Verification items for the finished model (mm, model axes). Face numbers are marked on the shaded views. A direction names the side the tool comes from. Round coordinates to 2 decimals unless told otherwise and drop trailing zeros. Loops run counter-clockwise (first coordinate to the right, second up) from the corner with the lowest first, then second, coordinate; pieces in that order, holes last. Notation, with made-up numbers: (82.25, 57) -> (88.25, 57) arc R22 ccw to (88.25, 63) -> close; hole circle Ø6 at (63.25, -12). An arc over 180 degrees is marked (long way). Write item = value, one per line.
```python
from build123d import *

# Parameters (mm, degrees)
BASE_FLANGE1_DEPTH      = 0.508
EDGE_FLANGE2_START      = -4.7625
EDGE_FLANGE2_DEPTH      = 9.525
EDGE_FLANGE2_2_DEPTH    = 9.525
EDGE_FLANGE3_START      = -4.7625
EDGE_FLANGE3_DEPTH      = 9.525
EDGE_FLANGE3_2_DEPTH    = 9.525
FILLET1_R               = 3.175
SKETCH17_R              = 1.8415
CUT_EXTRUDE1_DEPTH      = 23.441501951
EDGE_FLANGE4_DEPTH      = 4.445
EDGE_FLANGE4_BEND_DEPTH = 4.445
FILLET2_R               = 1.524
EDGE_FLANGE5_DEPTH      = 2.57875744
EDGE_FLANGE5_BEND_DEPTH = 2.57875744
FILLET3_R               = 0.762


# Read off the part's stored shape, not the designer's step: Edge-Flange2, Edge-Flange3
# Sheet-metal steps are written as plain solids
with BuildPart() as part:
    # Sketch1 → Base-Flange1 (new body)
    with BuildSketch(Plane(origin=(0, 0, 0), x_dir=(1, 0, 0), z_dir=(0, 1, 0))):
        with BuildLine():
            Line((-4.7625, -6.35), (-4.7625, -8.89))
            Line((-4.7625, -8.89), (4.7625, -8.89))
            Line((4.7625, -8.89), (4.7625, -6.35))
            ThreePointArc((4.7625, -6.35), (6.526150521, -4.518104207), (7.62, -2.2225))
            Line((7.62, -2.2225), (7.62, 2.2225))
            ThreePointArc((7.62, 2.2225), (6.526150521, 4.518104207), (4.7625, 6.35))
            Line((4.7625, 6.35), (4.7625, 8.89))
            Line((4.7625, 8.89), (-4.7625, 8.89))
            Line((-4.7625, 8.89), (-4.7625, 6.35))
            ThreePointArc((-4.7625, 6.35), (-6.526150521, 4.518104207), (-7.62, 2.2225))
            Line((-7.62, 2.2225), (-7.62, -2.2225))
            ThreePointArc((-7.62, -2.2225), (-6.526150521, -4.518104207), (-4.7625, -6.35))
        make_face()
    extrude(amount=-BASE_FLANGE1_DEPTH)

    # Edge-Flange2 outline → Edge-Flange2 (cut)
    with BuildSketch(Plane.YZ.offset(EDGE_FLANGE2_START)):
        with BuildLine():
            Line((0, -8.89), (0, -8.708309596))
            ThreePointArc((0, -8.708309596), (-0.373760644, -8.267342948), (-0.508, -7.70508998))
            Line((-0.508, -7.70508998), (-0.508, -8.89))
            Line((-0.508, -8.89), (0, -8.89))
        make_face()
    extrude(amount=EDGE_FLANGE2_DEPTH, mode=Mode.SUBTRACT)

    # Edge-Flange2 2 outline → Edge-Flange2 2 (add)
    with BuildSketch(Plane.YZ.offset(EDGE_FLANGE2_START)):
        with BuildLine():
            ThreePointArc((0, -8.708309596), (0.297808861, -8.869775128), (0.628125963, -8.944953901))
            Line((0.628125963, -8.944953901), (9.360304679, -9.708920547))
            Line((9.360304679, -9.708920547), (9.404579797, -9.20285364))
            Line((9.404579797, -9.20285364), (0.67240108, -8.438886994))
            ThreePointArc((0.67240108, -8.438886994), (0.193521514, -8.202729727), (0, -7.70508998))
            Line((0, -7.70508998), (0, -8.708309596))
        make_face()
    extrude(amount=EDGE_FLANGE2_2_DEPTH)

    # Edge-Flange3 outline → Edge-Flange3 (cut)
    with BuildSketch(Plane.YZ.offset(EDGE_FLANGE3_START)):
        with BuildLine():
            ThreePointArc((-0.508, 7.576201681), (-0.373760644, 8.138454649), (0, 8.579421297))
            Line((0, 8.579421297), (0, 8.89))
            Line((0, 8.89), (-0.508, 8.89))
            Line((-0.508, 8.89), (-0.508, 7.576201681))
        make_face()
    extrude(amount=EDGE_FLANGE3_DEPTH, mode=Mode.SUBTRACT)

    # Edge-Flange3 2 outline → Edge-Flange3 2 (add)
    with BuildSketch(Plane.YZ.offset(EDGE_FLANGE3_START)):
        with BuildLine():
            Line((10.878505399, 7.938254101), (0.845074037, 8.816065602))
            ThreePointArc((0.845074037, 8.816065602), (0.400987593, 8.774698018), (0, 8.579421297))
            Line((0, 8.579421297), (0, 7.576201681))
            ThreePointArc((0, 7.576201681), (0.238960253, 8.119280167), (0.80079892, 8.309998695))
            Line((0.80079892, 8.309998695), (10.834230282, 7.432187195))
            Line((10.834230282, 7.432187195), (10.878505399, 7.938254101))
        make_face()
    extrude(amount=EDGE_FLANGE3_2_DEPTH)

    # Fillet1
    fillet1_edges = [part.edges().sort_by_distance(p)[0] for p in [
        (4.7625, 9.382442238, -9.455887093),
        (-4.7625, 9.382442238, -9.455887093),
        (-4.7625, 10.85636784, 7.685220648),
        (4.7625, 10.85636784, 7.685220648),
    ]]
    fillet(fillet1_edges, radius=FILLET1_R)

    # Sketch17 → Cut-Extrude1 (cut, through all)
    with BuildSketch(Plane(origin=(0, 0.77186615, 8.822470462), x_dir=(1, 0, 0), z_dir=(0, 0.08715574274765484, 0.9961946980917459))):
        with Locations(Location((0, 7.18548753, 0), (0, 0, 270))):
            Circle(SKETCH17_R)
    extrude(amount=-CUT_EXTRUDE1_DEPTH, mode=Mode.SUBTRACT)

    # Edge-Flange4 section (across the edge) → Edge-Flange4 (add)
    with BuildSketch(Plane(origin=(-8.3566, 0, -2.2225), x_dir=(1, 0, 0), z_dir=(0, 0, 1))):
        with BuildLine():
            Line((-0.508, 0.7366), (-0.508, 4.572))
            Line((-0.508, 4.572), (0, 4.572))
            Line((0, 4.572), (0, 0.7366))
            ThreePointArc((0, 0.7366), (0.215745145, 0.215745145), (0.7366, 0))
            Line((0.7366, 0), (0.7366, -0.508))
            ThreePointArc((0.7366, -0.508), (-0.1434651, -0.1434651), (-0.508, 0.7366))
        make_face()
    extrude(amount=EDGE_FLANGE4_DEPTH)

    # Edge-Flange4 section 2 (across the edge) → Edge-Flange4 bend (add)
    with BuildSketch(Plane(origin=(8.3566, 0, 2.2225), x_dir=(-1, 0, 0), z_dir=(0, 0, -1))):
        with BuildLine():
            Line((-0.508, 0.7366), (-0.508, 4.572))
            Line((-0.508, 4.572), (0, 4.572))
            Line((0, 4.572), (0, 0.7366))
            ThreePointArc((0, 0.7366), (0.215745145, 0.215745145), (0.7366, 0))
            Line((0.7366, 0), (0.7366, -0.508))
            ThreePointArc((0.7366, -0.508), (-0.1434651, -0.1434651), (-0.508, 0.7366))
        make_face()
    extrude(amount=EDGE_FLANGE4_BEND_DEPTH)

    # Fillet2
    fillet2_edges = [part.edges().sort_by_distance(p)[0] for p in [
        (-8.6106, 4.572, -2.2225),
        (-8.6106, 4.572, 2.2225),
        (8.6106, 4.572, 2.2225),
        (8.6106, 4.572, -2.2225),
    ]]
    fillet(fillet2_edges, radius=FILLET2_R)

    # Edge-Flange5 section (across the edge) → Edge-Flange5 (add)
    with BuildSketch(Plane(origin=(-5.4991, 5.102367626, 7.933660198), x_dir=(1, 0, 0), z_dir=(0, 0.9961946980917459, -0.08715574274765468))):
        with BuildLine():
            Line((-0.508, 0.7366), (-0.508, 4.064))
            Line((-0.508, 4.064), (0, 4.064))
            Line((0, 4.064), (0, 0.7366))
            ThreePointArc((0, 0.7366), (0.215745145, 0.215745145), (0.7366, 0))
            Line((0.7366, 0), (0.7366, -0.508))
            ThreePointArc((0.7366, -0.508), (-0.1434651, -0.1434651), (-0.508, 0.7366))
        make_face()
    extrude(amount=EDGE_FLANGE5_DEPTH)

    # Edge-Flange5 section 2 (across the edge) → Edge-Flange5 bend (add)
    with BuildSketch(Plane(origin=(5.4991, 7.671312115, 7.708906678), x_dir=(-1, 0, 0), z_dir=(0, -0.9961946980917459, 0.08715574274765468))):
        with BuildLine():
            Line((-0.508, 0.7366), (-0.508, 4.064))
            Line((-0.508, 4.064), (0, 4.064))
            Line((0, 4.064), (0, 0.7366))
            ThreePointArc((0, 0.7366), (0.215745145, 0.215745145), (0.7366, 0))
            Line((0.7366, 0), (0.7366, -0.508))
            ThreePointArc((0.7366, -0.508), (-0.1434651, -0.1434651), (-0.508, 0.7366))
        make_face()
    extrude(amount=EDGE_FLANGE5_BEND_DEPTH)

    # Fillet3
    fillet3_edges = [part.edges().sort_by_distance(p)[0] for p in [
        (-5.7531, 4.748166688, 3.885124945),
        (-5.7531, 7.317111177, 3.660371425),
        (5.7531, 7.317111177, 3.660371425),
        (5.7531, 4.748166688, 3.885124945),
    ]]
    fillet(fillet3_edges, radius=FILLET3_R)


solid = part.part
```
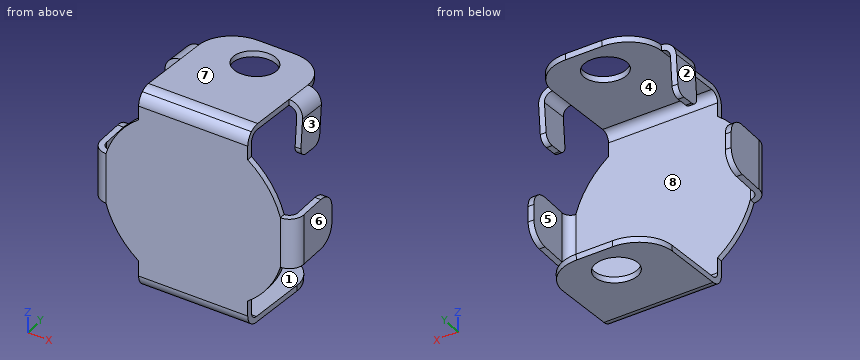
(1) Material ranges on probe 1 along X at (y, z) = (3.25, -0.75); probe 2 along Y at (x, z) = (3.5, -5); probe 3 along X at (y, z) = (6.25, 4.75), recorded low to high. Write a range as from..to.
Filled sheet:
probe_1 = -8.86..-8.36, 8.36..8.86
probe_2 = -0.51..0
probe_3 = -6.01..-5.5, 5.5..6.01
(2) Sectioned sample at B-B, the plane x = -0.75. Record the cut outline in (y, z).
Filled sheet:
outline = (-0.51, -7.71) arc R1.24 ccw to (0.63, -8.94) -> (4.71, -9.3) -> (4.76, -8.8) -> (0.67, -8.44) arc R0.74 cw to (0, -7.71) -> (0, 7.58) arc R0.74 cw to (0.8, 8.31) -> (6.21, 7.84) -> (6.25, 8.34) -> (0.85, 8.82) arc R1.24 ccw to (-0.51, 7.58) -> close; (8.06, -9.6) -> (9.36, -9.71) -> (9.4, -9.2) -> (8.11, -9.09) -> close; (9.56, 7.54) -> (10.83, 7.43) -> (10.88, 7.94) -> (9.61, 8.05) -> close
(3) Sectioned sample at A-A, the plane y = 1.5. Record the cut outline in (x, z), and give its area (3 significant figures).
Filled sheet:
outline = (-8.86, -2.22) -> (-8.36, -2.22) -> (-8.36, 2.22) -> (-8.86, 2.22) -> close; (-4.76, -9.02) -> (4.76, -9.02) -> (4.76, -8.51) -> (-4.76, -8.51) -> close; (-4.76, 8.25) -> (4.76, 8.25) -> (4.76, 8.76) -> (-4.76, 8.76) -> close; (8.36, -2.22) -> (8.86, -2.22) -> (8.86, 2.22) -> (8.36, 2.22) -> close
area = 14.2 mm2
(4) Sectioned sample at C-C, the plane z = -7. Record the cut outline in (x, y).
Filled sheet:
outline = (-4.76, -0.51) -> (4.76, -0.51) -> (4.76, 0) -> (-4.76, 0) -> close
(5) Go/stop test with flat-tipped pins: pin 1 Ø1.4 at (y, z) = (6, 5) entering from +X; pin 2 Ø0.6 at (x, y) = (-8, 1.5) entering from +Z (1 decimal); pin 3 Ø0.6 at (x, z) = (-8.5, 0) entering from +Y; pin 4 Ø1.4 at (y, z) = (6.5, 5) entering from -X. Record where each tip stops, or that it passes through.
Filled sheet:
pin_1 = 6.01
pin_2 = through
pin_3 = 4.57
pin_4 = -6.01
(6) Sectioned sample at D-D, the plane x = -4.25. Record the cut outline in (y, z).
Filled sheet:
outline = (-0.51, -7.71) arc R1.24 ccw to (0.63, -8.94) -> (7.92, -9.58) -> (7.96, -9.08) -> (0.67, -8.44) arc R0.74 cw to (0, -7.71) -> (0, 7.58) arc R0.74 cw to (0.8, 8.31) -> (9.39, 7.56) -> (9.44, 8.06) -> (0.85, 8.82) arc R1.24 ccw to (-0.51, 7.58) -> close
(7) Draft check along Z on the marked faces 6, 7 and 8. Enter one of: released by +Z, released by -Z, zero draft, split by the parting line, or undercut.
Filled sheet:
face_6 = zero draft
face_7 = released by +Z
face_8 = undercut
(8) Set-up check for the marked faces 1, 2, 3, 4 and 5: record each of +Z, -Z, +X, -X, +Y, -Y from which the full face is reachable in a straight line by a thin tool's end or side.
Filled sheet:
face_1 = +X, -X, +Y
face_2 = +Z, -Z, -X, +Y
face_3 = +Z, -Z, +X, +Y
face_4 = none
face_5 = +Z, -Z, +Y
